The figure shows three views and two pictorial views of one solid part (mm, origin at its lowest corner). Answer the questions. A direction names the side the tool comes from. Give positions to 0.01 mm unless a question says otherwise; leave off trailing zeros. Order: outer loops, then holes, each group sorted by start corner. A loop starts at its lowest first (then second) coordinate and runs counter-clockwise, first axis right, second up. Notation, with made-up numbers: (-25, 64.25) - (2, 64.25) arc R20 cw to (2, 93.25) - close; hole circle Ø10 at (-36.5, -20.5). An arc over 180 degrees is marked (long way). Answer as a JSON object with one key per item and string values. Group by question number.
Q1. Given pin 1 (5 mm diameter, centred on y = 5.5, z = 19.5, fed in from -X); pin 2 (5 mm diameter, centred on x = 47.5, y = 31, fed in from +Z); pin 3 (5 mm diameter, centred on y = 5, z = 24.5, fed in from +X), each flat-ended and moving along its own axis, determine where each tip first touches the part or whether it passes through.
Q2. A cutting plane is placed at C-C, the plane z = 27.5. Give the vertices of the cut face in (x, y).
Q3. A cutting plane is placed at D-D, the plane x = 73.5. Give the vertices of the cut face in (y, z).
Q4. For the marked faces 1, 2, 3, 4 and 5, determine the directions among +Z, -Z, +X, -X, +Y, -Y from which every point of the face is accessible in a straight line to the end or side of a thin tool.
Q5. Consider line 1 (Y direction, x = 45.5, z = 34.5); line 2 (X direction, y = 2.75, z = 27.5); line 3 (Z direction, x = 5.5, y = 34). Determine where each line is inside the solid, lowest interval first.
Q6. The mould has two halves that part along Y. Classify the marked faces 6, 7 and 8: released by +Y, released by -Y, zero draft, split by the parting line, or undercut.
Q7. A cutting plane is placed at A-A, the plane x = 45. Give the vertices of the cut face in (y, z).
Q8. A cutting plane is placed at B-B, the plane y = 6. Give the vertices of the cut face in (x, z), and give its area (3 significant figures).
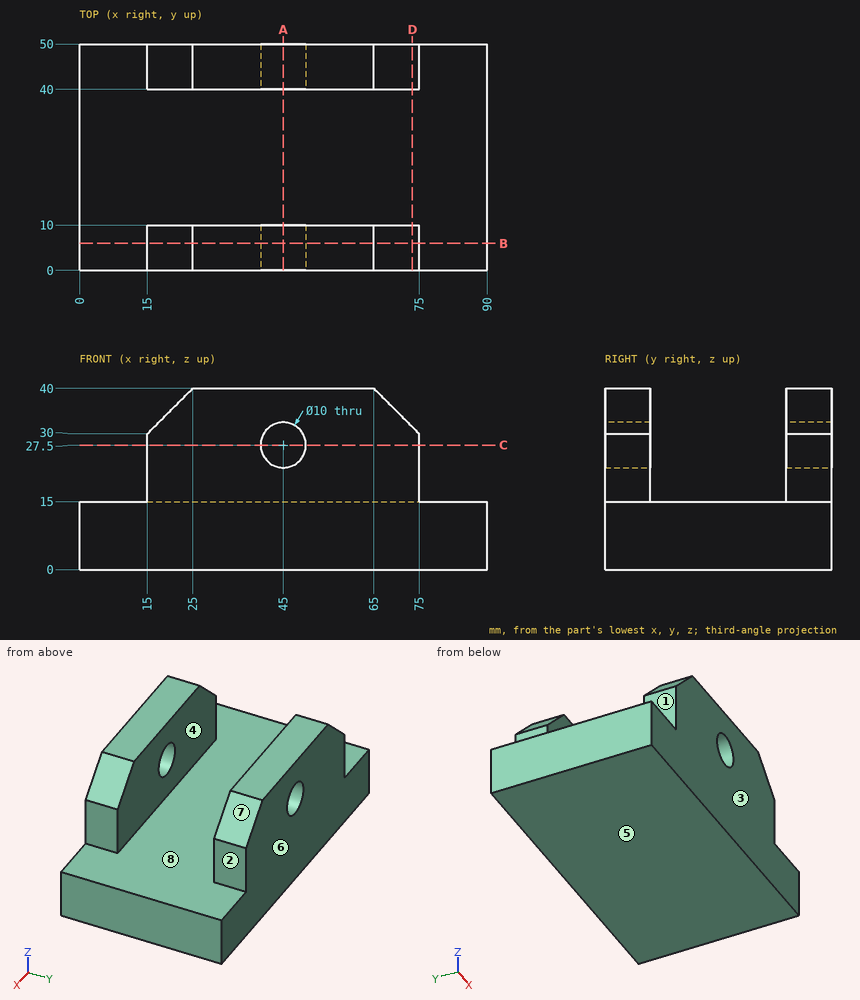
Reply:
{
 "1": {"pin 1": "stops at x = 15", "pin 2": "stops at z = 15", "pin 3": "stops at x = 75"},
 "2": {"outline": "(15, 0) - (40, 0) - (40, 10) - (15, 10) - close; (15, 40) - (40, 40) - (40, 50) - (15, 50) - close; (50, 0) - (75, 0) - (75, 10) - (50, 10) - close; (50, 40) - (75, 40) - (75, 50) - (50, 50) - close"},
 "3": {"outline": "(0, 0) - (50, 0) - (50, 31.5) - (40, 31.5) - (40, 15) - (10, 15) - (10, 31.5) - (0, 31.5) - close"},
 "4": {"face 1": "+Z, -X, +Y, -Y", "face 2": "+Z, +X, +Y, -Y", "face 3": "+Z, -Z, +X, -X, -Y", "face 4": "+Z, +X, -X", "face 5": "-Z, +X, -X, +Y, -Y"},
 "5": {"line 1": "y = 0 to 10, 40 to 50", "line 2": "x = 15 to 40, 50 to 75", "line 3": "z = 0 to 15"},
 "6": {"face 6": "released by +Y", "face 7": "zero draft", "face 8": "undercut"},
 "7": {"outline": "(0, 0) - (50, 0) - (50, 22.5) - (40, 22.5) - (40, 15) - (10, 15) - (10, 22.5) - (0, 22.5) - close; (0, 32.5) - (10, 32.5) - (10, 40) - (0, 40) - close; (40, 32.5) - (50, 32.5) - (50, 40) - (40, 40) - close"},
 "8": {"outline": "(0, 0) - (90, 0) - (90, 15) - (75, 15) - (75, 30) - (65, 40) - (25, 40) - (15, 30) - (15, 15) - (0, 15) - close; hole circle Ø10 at (45, 27.5)", "area": "2,670 mm^2"}
}
